Input: part model. Units: mm. Frame: model coordinates. Face numbers are marked on the shaded views. A direction names the side the tool comes from. Round coordinates to 2 decimals unless told otherwise and drop trailing zeros. Loops run counter-clockwise (first coordinate to the right, second up) from the corner with the lowest first, then second, coordinate; pieces in that order, holes last. Notation, with made-up numbers: (64, 60) - (94, 60) arc R15 cw to (94, 84) - close; hole circle Ø7 at (49.5, 66.25). An arc over 180 degrees is marked (long way). Write each question's results on one line, items separated by ' | '.
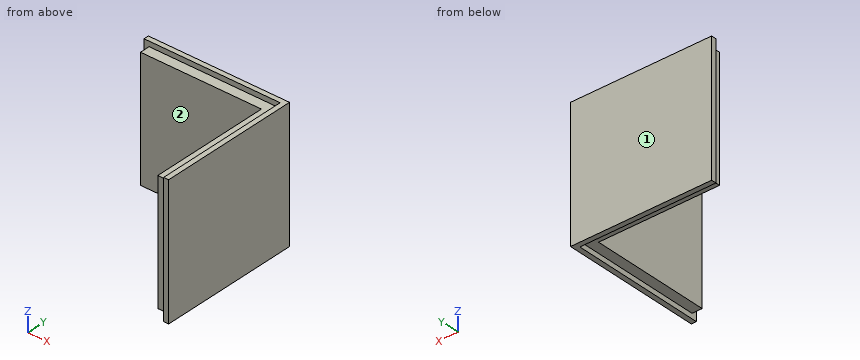
from build123d import *

# Parameters (mm, degrees)
SALIENTE_EXTRUIR1_DEPTH = 65
SALIENTE_EXTRUIR2_DEPTH = 60


with BuildPart() as part:
    # Croquis1 → Saliente-Extruir1 (new, symmetric)
    with BuildSketch(Plane.XY):
        Polygon((-70, 72.5), (70, 72.5), (70, -67.5), (65, -67.5), (65, 67.5), (-70, 67.5), align=None)
    extrude(amount=SALIENTE_EXTRUIR1_DEPTH, both=True)

    # Croquis2 → Saliente-Extruir2 (add, symmetric)
    with BuildSketch(Plane.XY):
        Polygon((-65, 67.5), (-65, 57.5), (55, 57.5), (55, -62.5), (65, -62.5), (65, 67.5), align=None)
    extrude(amount=SALIENTE_EXTRUIR2_DEPTH, both=True)


solid = part.part
1. Section query B-B, the plane y = 14.5. Output: boundary loops of the cut face in (x, z), plus the area to 3 significant figures.
Answer:
outline: (55, -60) - (65, -60) - (65, -65) - (70, -65) - (70, 65) - (65, 65) - (65, 60) - (55, 60) - close | area: 1,850 mm^2
2. Contact query for flat-ended pins moving along their axis: pin 1 (1.5 mm diameter, centred on x = -34, z = 8.5, fed in from -Y); pin 2 (5 mm diameter, centred on y = 63, z = -26, fed in from -X); pin 3 (8 mm diameter, centred on x = 58.5, z = 19.5, fed in from -Y). Output: stop coordinate, or through.
Answer:
pin 1: y = 57.5 | pin 2: x = -65 | pin 3: y = -62.5
3. Set-up query: the marked faces 1 and 2. Return all of +Z, -Z, +X, -X, +Y, -Y with unobstructed straight access to the full face (end or side cutting, diameter ignored); none if empty.
Answer:
face 1: +Z, -Z, +X, -X, +Y | face 2: +Z, -Z, -X, -Y
4. Section query A-A, the plane x = -20. Output: boundary loops of the cut face in (y, z), plus the area to 3 significant figures.
Answer:
outline: (57.5, -60) - (67.5, -60) - (67.5, -65) - (72.5, -65) - (72.5, 65) - (67.5, 65) - (67.5, 60) - (57.5, 60) - close | area: 1,850 mm^2
5. Section query C-C, the plane z = -56. Output: boundary loops of the cut face in (x, y), plus the area to 4 significant figures.
Answer:
outline: (-70, 67.5) - (-65, 67.5) - (-65, 57.5) - (55, 57.5) - (55, -62.5) - (65, -62.5) - (65, -67.5) - (70, -67.5) - (70, 72.5) - (-70, 72.5) - close | area: 3,875 mm^2
6. Line query: line 1 (X direction, y = -13, z = -48); line 2 (Y direction, x = 27, z = -55); line 3 (X direction, y = 61, z = 42.5). Output: solid intervals per line, ascending. Write a range as [from, to].
Answer:
line 1: [55, 70] | line 2: [57.5, 72.5] | line 3: [-65, 70]
